from build123d import *

# Parameters (mm, degrees)
SKETCH_1_R          = 1.5
EXTRUDE_1_DEPTH     = 6.7
SKETCH_2_W          = 19.1
SKETCH_2_H          = 29
EXTRUDE_2_DEPTH     = 2
CUT_EXTRUDE_1_REACH = 80.518
SKETCH_3_R          = 3.5
FILLET_1_R          = 0.4


with BuildPart() as part:
    # 草图1 → 凸台-拉伸1 (new body)
    with BuildSketch(Plane(origin=(0, 0, 0), x_dir=(0, 0, -1), z_dir=(1, 0, 0))):
        with BuildLine():
            Line((5, 0), (53, 0))
            ThreePointArc((53, 0), (56.535533906, -1.464466094), (58, -5))
            Line((58, -5), (58, -47.5))
            ThreePointArc((58, -47.5), (56.535533906, -51.035533906), (53, -52.5))
            Line((53, -52.5), (5, -52.5))
            ThreePointArc((5, -52.5), (1.464466094, -51.035533906), (0, -47.5))
            Line((0, -47.5), (0, -5))
            ThreePointArc((0, -5), (1.464466094, -1.464466094), (5, 0))
        make_face()
        with Locations((9, -8)):
            Circle(SKETCH_1_R, mode=Mode.SUBTRACT)
        with Locations((49, -8)):
            Circle(SKETCH_1_R, mode=Mode.SUBTRACT)
        with Locations((49, -44.5)):
            Circle(SKETCH_1_R, mode=Mode.SUBTRACT)
        with Locations((9, -44.5)):
            Circle(SKETCH_1_R, mode=Mode.SUBTRACT)
        with BuildLine():
            Line((5, -40.75), (22.1, -40.75))
            ThreePointArc((22.1, -40.75), (22.807106781, -40.457106781), (23.1, -39.75))
            Line((23.1, -39.75), (23.1, -12.75))
            ThreePointArc((23.1, -12.75), (22.807106781, -12.042893219), (22.1, -11.75))
            Line((22.1, -11.75), (5, -11.75))
            ThreePointArc((5, -11.75), (4.292893219, -12.042893219), (4, -12.75))
            Line((4, -12.75), (4, -39.75))
            ThreePointArc((4, -39.75), (4.292893219, -40.457106781), (5, -40.75))
        make_face(mode=Mode.SUBTRACT)
        with BuildLine():
            Line((53, -11.75), (35.9, -11.75))
            ThreePointArc((35.9, -11.75), (35.192893219, -12.042893219), (34.9, -12.75))
            Line((34.9, -12.75), (34.9, -39.75))
            ThreePointArc((34.9, -39.75), (35.192893219, -40.457106781), (35.9, -40.75))
            Line((35.9, -40.75), (53, -40.75))
            ThreePointArc((53, -40.75), (53.707106781, -40.457106781), (54, -39.75))
            Line((54, -39.75), (54, -12.75))
            ThreePointArc((54, -12.75), (53.707106781, -12.042893219), (53, -11.75))
        make_face(mode=Mode.SUBTRACT)
    extrude(amount=EXTRUDE_1_DEPTH)

    # 草图2 → 凸台-拉伸2 (add)
    with BuildSketch(Plane.ZY):
        with Locations((-13.55, -26.25)):
            Rectangle(SKETCH_2_W, SKETCH_2_H)
        with Locations((-44.45, -26.25)):
            Rectangle(SKETCH_2_W, SKETCH_2_H)
    extrude(amount=-EXTRUDE_2_DEPTH)

    # 草图3 → 切除-拉伸1 (cut, up to next)
    with BuildSketch(Plane(origin=(6.7, 0, 0), x_dir=(0, 0, -1), z_dir=(1, 0, 0)), mode=Mode.PRIVATE) as cut_extrude_1_sk1:
        with Locations((29, -26.25)):
            Circle(SKETCH_3_R)
    cut_extrude_1_tool1 = extrude(cut_extrude_1_sk1.sketch, amount=-CUT_EXTRUDE_1_REACH, mode=Mode.PRIVATE) & part.part
    add(cut_extrude_1_tool1.solids().sort_by_distance((6.7, -26.25, -29))[0], mode=Mode.SUBTRACT)

    # 圆角1
    fillet_1_edges = [part.edges().sort_by_distance(p)[0] for p in [
        (2, -26.25, -4),
        (2, -40.75, -13.55),
        (2, -26.25, -23.1),
        (2, -12.042893219, -4.292893219),
        (2, -40.457106781, -4.292893219),
        (2, -40.457106781, -22.807106781),
        (2, -12.042893219, -22.807106781),
        (2, -26.25, -34.9),
        (2, -40.75, -44.45),
        (2, -26.25, -54),
        (2, -11.75, -44.45),
        (2, -40.457106781, -35.192893219),
        (2, -40.457106781, -53.707106781),
        (2, -12.042893219, -53.707106781),
        (2, -12.042893219, -35.192893219),
        (2, -11.75, -13.55),
    ]]
    fillet(fillet_1_edges, radius=FILLET_1_R)


solid = part.part
Model file for the job. Use its own axes, mm. A direction names the side the tool comes from. Round coordinates to 2 decimals unless told otherwise and drop trailing zeros. Loops run counter-clockwise (first coordinate to the right, second up) from the corner with the lowest first, then second, coordinate; pieces in that order, holes last.
1. Band-saw the part on A-A, the plane z = -29. List the corners of the cut face in (x, y), and give its area (3 significant figures).
Check values:
outline: (0, -52.5) - (6.7, -52.5) - (6.7, -29.75) - (0, -29.75) - close; (0, -22.75) - (6.7, -22.75) - (6.7, 0) - (0, 0) - close
area: 305 mm2
2. Drop flat-ended pins along their axis: P1, Ø2, axis at y = -13, z = -21.5, coming from the -X side; P2, Ø5.5, axis at y = -25, z = -47.5, coming from the +X side. Give the stop position or say it passes through.
Check values:
P1: stops at x = 0
P2: stops at x = 2
3. Band-saw the part on B-B, the plane x = 4.75. Count the separate pieces of the cut face and the enclosed holes in it, and give its area (3 significant figures).
Check values:
separate pieces: 1
enclosed holes: 7
area: 1,850 mm2
4. Wall check: probe 1 along Z at (x, y) = (4.25, -33.5); probe 2 along Y at (x, z) = (4, -49); probe 3 along Y at (x, z) = (1.75, -49). Give the ranges that are in metal, low to high.
Check values:
probe 1: z = -58 to -54, -34.9 to -23.1, -4 to 0
probe 2: y = -52.5 to -46, -43 to -40.75, -11.75 to -9.5, -6.5 to 0
probe 3: y = -52.5 to -46, -43 to -9.5, -6.5 to 0
5. Mould opens along Y. For faces 3 (the flat face through (6.7, -32, -29)), 4 (the flat face through (3, -52.5, -29)), 5 (the flat face through (5, -26, -23.1)) say: +Y half, -Y half, draft (parallel to the pull), parting line (faces both ways), or undercut.
Check values:
face 3: draft
face 4: -Y half
face 5: undercut
6. Band-saw the part on D-D, the plane z = -9. List the corners of the cut face in (x, y), and give its area (3 significant figures).
Check values:
outline: (0, -52.5) - (6.7, -52.5) - (6.7, -46) - (0, -46) - close; (0, -43) - (6.7, -43) - (6.7, -40.75) - (2.4, -40.75) arc R0.4 cw to (2, -40.35) - (2, -12.15) arc R0.4 cw to (2.4, -11.75) - (6.7, -11.75) - (6.7, -9.5) - (0, -9.5) - close; (0, -6.5) - (6.7, -6.5) - (6.7, 0) - (0, 0) - close
area: 175 mm2
7. Tool access for faces 1 (the cylindrical face through (3.303, -9.464, -8.675)), 2 (the flat face through (5, -26, -54)): list every direction of +Z, -Z, +X, -X, +Y, -Y with a clear straight run to the whole face (end or side of a thin tool).
Check values:
face 1: +X, -X
face 2: +X
8. Band-saw the part on C-C, the plane y = -26.25. List the corners of the cut face in (x, z), and give its area (3 significant figures).
Check values:
outline: (0, -58) - (6.7, -58) - (6.7, -54) - (2.4, -54) arc R0.4 cw to (2, -53.6) - (2, -35.3) arc R0.4 cw to (2.4, -34.9) - (6.7, -34.9) - (6.7, -32.5) - (0, -32.5) - close; (0, -25.5) - (6.7, -25.5) - (6.7, -23.1) - (2.4, -23.1) arc R0.4 cw to (2, -22.7) - (2, -4.4) arc R0.4 cw to (2.4, -4) - (6.7, -4) - (6.7, 0) - (0, 0) - close
area: 162 mm2
